```python
from build123d import *

# Parameters (mm, degrees)
SKETCH1_W                       = 127
SKETCH1_H                       = 127
SKETCH1_R                       = 6.35
BOSS_EXTRUDE1_DEPTH             = 10.16
SKETCH3_R                       = 57.15
CUT_EXTRUDE1_DEPTH              = 6.35
BOSS_EXTRUDE2_REACH             = 181.717
SKETCH4_R                       = 6.35
BOSS_EXTRUDE2_DIRECTION_2_REACH = 181.717
SKETCH5_R                       = 3.175
CUT_EXTRUDE2_DEPTH              = 180.89226109


with BuildPart() as part:
    # Sketch1 → Boss-Extrude1 (new body)
    with BuildSketch(Plane.XY):
        with Locations((63.5, 63.5)):
            Rectangle(SKETCH1_W, SKETCH1_H)
        with Locations((90.440768363, 90.440768363)):
            Circle(SKETCH1_R, mode=Mode.SUBTRACT)
        with Locations((90.440768363, 36.559231637)):
            Circle(SKETCH1_R, mode=Mode.SUBTRACT)
        with BuildLine():
            ThreePointArc((36.020411647, 90.979588353), (24.637993463, 63.5), (36.020411647, 36.020411647))
            ThreePointArc((36.020411647, 36.020411647), (46.078298503, 36.020411647), (46.078298503, 46.078298503))
            ThreePointArc((46.078298503, 46.078298503), (38.861993463, 63.5), (46.078298503, 80.921701497))
            ThreePointArc((46.078298503, 80.921701497), (46.078298503, 90.979588353), (36.020411647, 90.979588353))
        make_face(mode=Mode.SUBTRACT)
    extrude(amount=BOSS_EXTRUDE1_DEPTH)

    # Sketch3 → Cut-Extrude1 (cut)
    with BuildSketch(Plane.XY.offset(10.16)):
        with Locations((63.5, 63.5)):
            Circle(SKETCH3_R)
    extrude(amount=-CUT_EXTRUDE1_DEPTH, mode=Mode.SUBTRACT)

    # Boss-Extrude2: up to this face of the body (flat: up to its plane)
    boss_extrude2_end = Plane(part.part.faces().sort_by_distance((63.5, 1.796051224, 10.16))[0])
    # Sketch4 → Boss-Extrude2 (add, up to the picked face)
    with BuildSketch(Plane.XY.offset(3.81), mode=Mode.PRIVATE) as boss_extrude2_sk1:
        with Locations(Location((90.440768363, 36.559231637, 0), (0, 0, 180))):
            Circle(SKETCH4_R)
    boss_extrude2_tool1 = split(extrude(boss_extrude2_sk1.sketch, amount=BOSS_EXTRUDE2_REACH, mode=Mode.PRIVATE), bisect_by=boss_extrude2_end, keep=Keep.BOTH, mode=Mode.PRIVATE)
    # Sketch4 → Boss-Extrude2 (add, up to the picked face)
    with BuildSketch(Plane.XY.offset(3.81), mode=Mode.PRIVATE) as boss_extrude2_sk2:
        with Locations(Location((90.440768363, 90.440768363, 0), (0, 0, 180))):
            Circle(SKETCH4_R)
    boss_extrude2_tool2 = split(extrude(boss_extrude2_sk2.sketch, amount=BOSS_EXTRUDE2_REACH, mode=Mode.PRIVATE), bisect_by=boss_extrude2_end, keep=Keep.BOTH, mode=Mode.PRIVATE)
    # Sketch4 → Boss-Extrude2 (add, up to the picked face)
    with BuildSketch(Plane.XY.offset(3.81), mode=Mode.PRIVATE) as boss_extrude2_sk3:
        with BuildLine():
            ThreePointArc((46.078298503, 80.921701497), (38.861993463, 63.5), (46.078298503, 46.078298503))
            ThreePointArc((46.078298503, 46.078298503), (46.078298503, 36.020411647), (36.020411647, 36.020411647))
            ThreePointArc((36.020411647, 36.020411647), (24.637993463, 63.5), (36.020411647, 90.979588353))
            ThreePointArc((36.020411647, 90.979588353), (46.078298503, 90.979588353), (46.078298503, 80.921701497))
        make_face()
    boss_extrude2_tool3 = split(extrude(boss_extrude2_sk3.sketch, amount=BOSS_EXTRUDE2_REACH, mode=Mode.PRIVATE), bisect_by=boss_extrude2_end, keep=Keep.BOTH, mode=Mode.PRIVATE)
    add(boss_extrude2_tool1.solids().sort_by(Axis((90.440768, 36.559232, 3.81), (0, 0, 1)))[0])
    add(boss_extrude2_tool2.solids().sort_by(Axis((90.440768, 90.440768, 3.81), (0, 0, 1)))[0])
    add(boss_extrude2_tool3.solids().sort_by(Axis((36.037587, 63.5, 3.81), (0, 0, 1)))[0])

    # Boss-Extrude2 direction 2: up to this face of the body (flat: up to its plane)
    boss_extrude2_direction_2_end = Plane(part.part.faces().sort_by_distance((64.634104548, 63.5, 0))[0])
    # Sketch4 → Boss-Extrude2 direction 2 (add, up to the picked face)
    with BuildSketch(Plane.XY.offset(3.81), mode=Mode.PRIVATE) as boss_extrude2_direction_2_sk1:
        with Locations(Location((90.440768363, 36.559231637, 0), (0, 0, 180))):
            Circle(SKETCH4_R)
    boss_extrude2_direction_2_tool1 = split(extrude(boss_extrude2_direction_2_sk1.sketch, amount=-BOSS_EXTRUDE2_DIRECTION_2_REACH, mode=Mode.PRIVATE), bisect_by=boss_extrude2_direction_2_end, keep=Keep.BOTH, mode=Mode.PRIVATE)
    # Sketch4 → Boss-Extrude2 direction 2 (add, up to the picked face)
    with BuildSketch(Plane.XY.offset(3.81), mode=Mode.PRIVATE) as boss_extrude2_direction_2_sk2:
        with Locations(Location((90.440768363, 90.440768363, 0), (0, 0, 180))):
            Circle(SKETCH4_R)
    boss_extrude2_direction_2_tool2 = split(extrude(boss_extrude2_direction_2_sk2.sketch, amount=-BOSS_EXTRUDE2_DIRECTION_2_REACH, mode=Mode.PRIVATE), bisect_by=boss_extrude2_direction_2_end, keep=Keep.BOTH, mode=Mode.PRIVATE)
    # Sketch4 → Boss-Extrude2 direction 2 (add, up to the picked face)
    with BuildSketch(Plane.XY.offset(3.81), mode=Mode.PRIVATE) as boss_extrude2_direction_2_sk3:
        with BuildLine():
            ThreePointArc((46.078298503, 80.921701497), (38.861993463, 63.5), (46.078298503, 46.078298503))
            ThreePointArc((46.078298503, 46.078298503), (46.078298503, 36.020411647), (36.020411647, 36.020411647))
            ThreePointArc((36.020411647, 36.020411647), (24.637993463, 63.5), (36.020411647, 90.979588353))
            ThreePointArc((36.020411647, 90.979588353), (46.078298503, 90.979588353), (46.078298503, 80.921701497))
        make_face()
    boss_extrude2_direction_2_tool3 = split(extrude(boss_extrude2_direction_2_sk3.sketch, amount=-BOSS_EXTRUDE2_DIRECTION_2_REACH, mode=Mode.PRIVATE), bisect_by=boss_extrude2_direction_2_end, keep=Keep.BOTH, mode=Mode.PRIVATE)
    add(boss_extrude2_direction_2_tool1.solids().sort_by(Axis((90.440768, 36.559232, 3.81), (0, 0, -1)))[0])
    add(boss_extrude2_direction_2_tool2.solids().sort_by(Axis((90.440768, 90.440768, 3.81), (0, 0, -1)))[0])
    add(boss_extrude2_direction_2_tool3.solids().sort_by(Axis((36.037587, 63.5, 3.81), (0, 0, -1)))[0])

    # Sketch5 → Cut-Extrude2 (cut, through all)
    with BuildSketch(Plane.XY.offset(10.16)):
        with Locations((90.440768363, 90.440768363)):
            Circle(SKETCH5_R)
        with Locations((90.440768363, 36.559231637)):
            Circle(SKETCH5_R)
    extrude(amount=-CUT_EXTRUDE2_DEPTH, mode=Mode.SUBTRACT)


solid = part.part
```
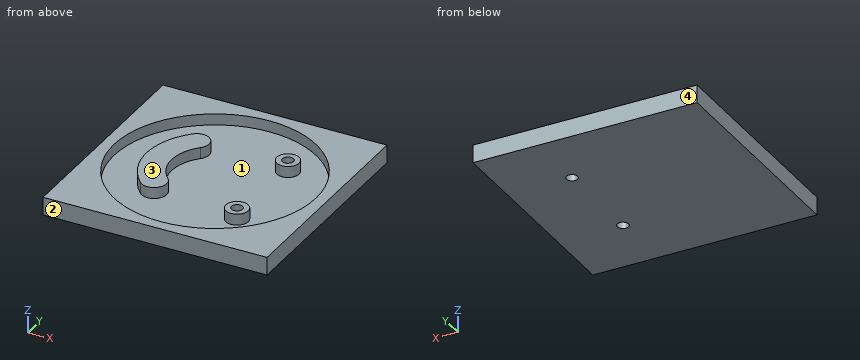
CAD build for the part. Positions are in the model's coordinates, mm. Face numbers are marked on the shaded views. Round coordinates to 2 decimals unless told otherwise and drop trailing zeros. Write each loop counter-clockwise with the first axis right and the second up, starting at its lowest first coordinate (ties: lowest second). Pieces come first, ordered by that corner, then holes. Notation, with made-up numbers: (0.5, -33.5) -> (7.5, -33.5) arc R24 ccw to (7.5, 0.5) -> close; hole circle Ø4 at (32.5, -23). An arc over 180 degrees is marked (long way). Answer in a Markdown table with one row per item. Add a question column.
Item 1: Saw through at D-D, the plane x = 91. Write the cut outline in (y, z), then the cut area to 3 significant figures.
Item 2: Saw through at B-B, the plane y = 63.5. Write the cut outline in (x, z), then the cut area to 3 significant figures.
Item 3: Saw through at C-C, the plane x = 63.5. Write the cut outline in (y, z).
Item 4: Drop a flat-ended pin along its axis: pin 1 Ø2 at (x, y) = (14.5, 66) entering from +Z. Give the stop position or say it passes through.
Item 5: Drill centre lines: line 1 (Y direction, x = 63.5, z = 7.25); line 2 (Y direction, x = 91.5, z = 4.25); line 3 (X direction, y = 60.5, z = 8.75). Where is each one in solid material? Low to high. Write a range as from..to.
Item 6: Saw through at A-A, the plane z = 7. Write the cut outline in (x, y) (3 decimals), then the cut area to 3 significant figures.
Item 7: Mould opens along Y. For the marked faces 1, 2, 3 and 4 say: pulls with the +Y half, pulls with the -Y half, needs draft (parallel to the pull), parting line crosses it, or undercut.
Findings below:
| question | item | result |
|---|---|---|
| 1 | outline | (0, 0) -> (33.43, 0) -> (33.43, 10.16) -> (30.23, 10.16) -> (30.23, 3.81) -> (13.4, 3.81) -> (13.4, 10.16) -> (0, 10.16) -> close; (39.68, 0) -> (87.32, 0) -> (87.32, 10.16) -> (84.12, 10.16) -> (84.12, 3.81) -> (42.88, 3.81) -> (42.88, 10.16) -> (39.68, 10.16) -> close; (93.57, 0) -> (127, 0) -> (127, 10.16) -> (113.6, 10.16) -> (113.6, 3.81) -> (96.77, 3.81) -> (96.77, 10.16) -> (93.57, 10.16) -> close |
| 1 | area | 688 mm^2 |
| 2 | outline | (0, 0) -> (127, 0) -> (127, 10.16) -> (120.65, 10.16) -> (120.65, 3.81) -> (38.86, 3.81) -> (38.86, 10.16) -> (24.64, 10.16) -> (24.64, 3.81) -> (6.35, 3.81) -> (6.35, 10.16) -> (0, 10.16) -> close |
| 2 | area | 655 mm^2 |
| 3 | outline | (0, 0) -> (127, 0) -> (127, 10.16) -> (120.65, 10.16) -> (120.65, 3.81) -> (6.35, 3.81) -> (6.35, 10.16) -> (0, 10.16) -> close |
| 4 | pin 1 | stops at z = 3.81 |
| 5 | line 1 | y = 0..6.35, 120.65..127 |
| 5 | line 2 | y = 0..13.68, 30.3..33.57, 39.55..42.82, 84.18..87.45, 93.43..96.7, 113.32..127 |
| 5 | line 3 | x = 0..6.43, 24.75..39.05, 120.57..127 |
| 6 | outline | (0, 0) -> (127, 0) -> (127, 127) -> (0, 127) -> close; (36.02, 36.02) arc R7.112 ccw to (46.078, 46.078) arc R24.638 cw to (46.078, 80.922) arc R7.112 ccw to (36.02, 90.98) arc R38.862 ccw to start; circle Ø12.7 at (90.441, 36.559); circle Ø12.7 at (90.441, 90.441); hole circle Ø114.3 at (63.5, 63.5); hole circle Ø6.35 at (90.441, 36.559); hole circle Ø6.35 at (90.441, 90.441) |
| 6 | area | 6,930 mm^2 |
| 7 | face 1 | undercut |
| 7 | face 2 | pulls with the -Y half |
| 7 | face 3 | needs draft |
| 7 | face 4 | pulls with the +Y half |
